```python
from build123d import *

# Parameters (mm, degrees)
ESBO_O1_R                  = 6.35
RESSALTO_EXTRUS_O1_DEPTH   = 200
ESBO_O2_R                  = 12.7
ESBO_O2_R_2                = 4
CORTE_EXTRUS_O1_DEPTH      = 201.201510983
CORTE_EXTRUS_O2_DEPTH      = 201.079984006
CORTE_EXTRUS_O2_DEPTH_BACK = 201.079984006
ESBO_O3_W                  = 12
ESBO_O3_H                  = 10
ESBO_O5_W                  = 12
ESBO_O5_H                  = 10


with BuildPart() as part:
    # Esboço1 → Ressalto-extrusão1 (new body)
    with BuildSketch(Plane.XY):
        Circle(ESBO_O1_R)
    extrude(amount=RESSALTO_EXTRUS_O1_DEPTH)

    # Esboço2 → Corte-extrusão1 (cut, through all)
    with BuildSketch(Plane.XY.offset(200)):
        Circle(ESBO_O2_R)
        Circle(ESBO_O2_R_2, mode=Mode.SUBTRACT)
    extrude(amount=-CORTE_EXTRUS_O1_DEPTH, mode=Mode.SUBTRACT)

    # Esboço3 → Corte-extrusão2 (cut, two sides: drawn at the far end of the back side and taken through both)
    with BuildSketch(Plane(origin=(0, 0, 0), x_dir=(0, 0, -1), z_dir=(1, 0, 0)).offset(-CORTE_EXTRUS_O2_DEPTH_BACK)):
        with Locations((-194, 7)):
            Rectangle(ESBO_O3_W, ESBO_O3_H)
    extrude(amount=CORTE_EXTRUS_O2_DEPTH + CORTE_EXTRUS_O2_DEPTH_BACK, mode=Mode.SUBTRACT)

    # Esboço5 → Corte-Revolução2 (revolve, cut)
    with BuildSketch(Plane(origin=(0, 0, 0), x_dir=(0, 0, -1), z_dir=(1, 0, 0)), mode=Mode.PRIVATE) as corte_revolu_o2_sk:
        with Locations((-194, 8)):
            Rectangle(ESBO_O5_W, ESBO_O5_H)
    revolve(corte_revolu_o2_sk.sketch.rotate(Axis((0, 0, 0), (0, 0, 1)), 270), axis=Axis((0, 0, 0), (0, 0, 1)), mode=Mode.SUBTRACT)


solid = part.part
```
Work out the finished part from the listing and answer in its coordinate system (mm). A direction names the side the tool comes from. Give positions to 0.01 mm unless a question says otherwise; leave off trailing zeros. Loops run counter-clockwise (first coordinate to the right, second up) from the corner with the lowest first, then second, coordinate; pieces in that order, holes last. Notation, with made-up numbers: (38, 66.5) -> (50, 66.5) arc R6 ccw to (50, 73.5) -> close; hole circle Ø6 at (-21, -20). An arc over 180 degrees is marked (long way). Put each result on its own line as item: value. Start each with the question number.
Item 1: Which of the six approach directions +Z, -Z, +X, -X, +Y, -Y give full straight-line access (tool end or side, diameter ignored) to faces 1 (the face through (0, 2, 194)), 2 (the face through (0, 0, 0)), 3 (the face through (0, -3, 194))?
Item 2: The part is cut by section B-B (z = 53.5). Give the vertices of the cut face in (x, y), then the cut area to 3 significant figures.
Item 3: Find the intervals of material crossed by L1, parallel to Y at x = 0.25, z = 80; L2, parallel to X at y = -0.5, z = 107; L3, parallel to Z at x = 3, y = 1.25, in increasing order. Write a range as [from, to].
Item 4: This flat-tipped pin is pushed along its axis until it touches: P1, Ø1.3, axis at x = -1, z = 194, coming from the +Y side. Where does it stop, or does it pass through?
Item 5: The part is cut by section A-A (x = 0). Give the vertices of the cut face in (y, z).
Answers below:
1. face 1: +Z, +X, -X, +Y
1. face 2: -Z, +X, -X, +Y, -Y
1. face 3: +Z
2. outline: circle Ø8 at (0, 0)
2. area: 50.3 mm2
3. L1: [-3.99, 3.99]
3. L2: [-3.97, 3.97]
3. L3: [0, 188]
4. P1: y = 2
5. outline: (-4, 0) -> (4, 0) -> (4, 188) -> (2, 188) -> (2, 200) -> (-3, 200) -> (-3, 188) -> (-4, 188) -> close
